Answer from the drawing. Dimensions are ordinates in mm from the lowest x, y and z of the part. A direction names the side the tool comes from. Coordinates: 2 decimals unless noted, no trailing zeros. Loops run counter-clockwise (first coordinate to the right, second up) from the corner with the lowest first, then second, coordinate; pieces in that order, holes last. Notation, with made-up numbers: M -26.5,63 L -8.5,63 A26 cw -8.5,95 Z; hole C 1.25,38.5 d3. An arc over 180 degrees is marked long. One line per item, written item: value. Start each with the question number.
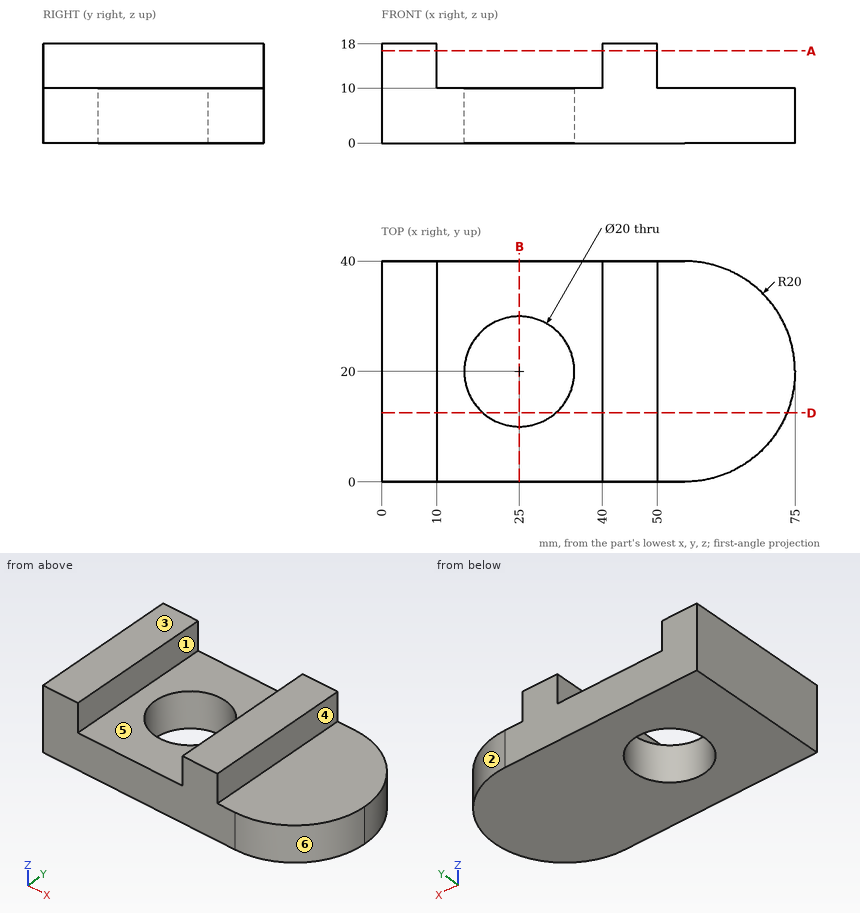
1) Section A-A (z = 16.75) is taken. Determine the outline of the cut face in (x, y).
2) For a pull along X with two mould halves and no side action, classify the marked faces 1, 2 and 3 as released by +X, released by -X, zero draft, split by the parting line, or undercut.
3) Section D-D (y = 12.5) is taken. Determine the outline of the cut face in (x, z).
4) A tool of negligible diameter and unlimited length cuts with its end or side. For the marked faces 4, 5 and 6, from which of +Z, -Z, +X, -X, +Y, -Y can it reach the whole face along a straight path? Write none if from no direction.
5) Section B-B (x = 25) is taken. Determine the outline of the cut face in (y, z), then the cut area to 3 significant figures.
6) Flat-ended cylindrical pins translate along their axes: pin 1 (1.5 mm diameter, centred on x = 37, z = 12.5, fed in from +Y) (3 decimals); pin 2 (12 mm diameter, centred on x = 23.5, y = 6, fed in from +Z); pin 3 (2.5 mm diameter, centred on y = 27.5, z = 12.5, fed in from +X); pin 4 (2 mm diameter, centred on x = 67, z = 2.5, fed in from +Y). Find the tip coordinate at first contact, or state that the pin passes through.
7) Consider line 1 along Y through (x, z) = (25, 7); line 2 along X through (y, z) = (25.5, 15); line 3 along Z through (x, y) = (25.5, 37). Determine where each line is inside the solid, lowest interval first.
Results found:
1. outline: M 0,0 L 10,0 L 10,40 L 0,40 Z; M 40,0 L 50,0 L 50,40 L 40,40 Z
2. face 1: undercut
2. face 2: released by +X
2. face 3: zero draft
3. outline: M 0,0 L 18.39,0 L 18.39,10 L 10,10 L 10,18 L 0,18 Z; M 31.61,0 L 73.54,0 L 73.54,10 L 50,10 L 50,18 L 40,18 L 40,10 L 31.61,10 Z
4. face 4: +Z, +X, +Y, -Y
4. face 5: +Z, +Y, -Y
4. face 6: +Z, -Z, +X, -Y
5. outline: M 0,0 L 10,0 L 10,10 L 0,10 Z; M 30,0 L 40,0 L 40,10 L 30,10 Z
5. area: 200 mm²
6. pin 1: passes through
6. pin 2: stops at z = 10
6. pin 3: stops at x = 50
6. pin 4: stops at y = 36.7
7. line 1: y = 0 to 10, 30 to 40
7. line 2: x = 0 to 10, 40 to 50
7. line 3: z = 0 to 10
